from build123d import *

# Parameters (mm, degrees)
SKETCH_1_W             = 60
SKETCH_1_H             = 60
EXTRUDE_1_DEPTH        = 12
HOLE_WIZARD_M141_D     = 12
HOLE_WIZARD_M141_DEPTH = 12
SKETCH_12_R            = 4.5
CUT_EXTRUDE_1_DEPTH    = 13
SKETCH_13_R            = 7.5
CUT_EXTRUDE_2_DEPTH    = 9


with BuildPart() as part:
    # Эскиз1 → Бобышка-Вытянуть1 (new body)
    with BuildSketch(Plane(origin=(0, 0, 0), x_dir=(1, 0, 0), z_dir=(0, 1, 0))):
        Rectangle(SKETCH_1_W, SKETCH_1_H)
    extrude(amount=EXTRUDE_1_DEPTH)

    # Отверстие обработанное метчиком M141
    with Locations(Plane(origin=(0, 12, 0), x_dir=(1, 0, 0), z_dir=(0, 1, 0))):
        with Locations((0, 0)):
            Hole(HOLE_WIZARD_M141_D / 2, depth=HOLE_WIZARD_M141_DEPTH)

    # Эскиз12 → Вырез-Вытянуть1 (cut, through all)
    with BuildSketch(Plane(origin=(0, 12, 0), x_dir=(1, 0, 0), z_dir=(0, 1, 0))):
        with Locations(Location((-15, 15, 0), (0, 0, 270))):  # turned: the seam where the file's is
            Circle(SKETCH_12_R)
        with Locations(Location((15, 15, 0), (0, 0, 270))):  # turned: the seam where the file's is
            Circle(SKETCH_12_R)
        with Locations(Location((15, -15, 0), (0, 0, 270))):  # turned: the seam where the file's is
            Circle(SKETCH_12_R)
        with Locations(Location((-15, -15, 0), (0, 0, 270))):  # turned: the seam where the file's is
            Circle(SKETCH_12_R)
    extrude(amount=-CUT_EXTRUDE_1_DEPTH, mode=Mode.SUBTRACT)

    # Эскиз13 → Вырез-Вытянуть2 (cut)
    with BuildSketch(Plane(origin=(0, 12, 0), x_dir=(1, 0, 0), z_dir=(0, 1, 0))):
        with Locations(Location((-15, 15, 0), (0, 0, 270))):  # turned: the seam where the file's is
            Circle(SKETCH_13_R)
        with Locations(Location((15, 15, 0), (0, 0, 270))):  # turned: the seam where the file's is
            Circle(SKETCH_13_R)
        with Locations(Location((15, -15, 0), (0, 0, 270))):  # turned: the seam where the file's is
            Circle(SKETCH_13_R)
        with Locations(Location((-15, -15, 0), (0, 0, 270))):  # turned: the seam where the file's is
            Circle(SKETCH_13_R)
    extrude(amount=-CUT_EXTRUDE_2_DEPTH, mode=Mode.SUBTRACT)


solid = part.part
The model under review builds one solid part; all positions refer to its coordinate system, in mm. A direction names the side the tool comes from. Give positions to 0.01 mm unless a question says otherwise; leave off trailing zeros. Order: outer loops, then holes, each group sorted by start corner. A loop starts at its lowest first (then second) coordinate and runs counter-clockwise, first axis right, second up. Notation, with made-up numbers: M 66.25,-35.75 L 91.25,-35.75 A12 cw 91.25,-14.75 Z; hole C -2.5,18.25 d3. An arc over 180 degrees is marked long. Answer in a Markdown table with one row per item. Add a question column.
1. To check wall thickness, follow line 1 along X through (y, z) = (4.75, -15); line 2 along X through (y, z) = (1.8, 15); line 3 along Z through (x, y) = (-20, 10.5). State the ranges of each line that lie inside material, in increasing order.
2. Add section A-A on z = -15. State the section outline as (x, y) points, plus the area to 3 significant figures.
3. Mouldability with a two-part tool opening along X and no side actions: class faces 3 (the cylindrical face through (-11.96, 1.52, -18.32)), 4 (the flat face through (-30, 6, 0)), 5 (the flat face through (30, 6, 0)) as released by +X, released by -X, zero draft, split by the parting line, or undercut.
4. Machinability: for faces 1 (the cylindrical face through (15.33, 7.563, -22.493)), 2 (the flat face through (-7, 12, 0)), which of the approach directions +Z, -Z, +X, -X, +Y, -Y give a long, thin tool a straight path to every point of the face, cutting with its end or side? Answer none if there is none.
5. Add section D-D on z = 4. State the section outline as (x, y) points, plus the area to 3 significant figures.
6. For pin 1 Ø13.5 at (x, z) = (-15, -15) entering from +Y, flat-tipped, find the tip position at first contact; note if it passes through.
7. Add section B-B on y = 1.75. State the section outline as (x, z) points.
8. Add section C-C on x = 13. State the section outline as (y, z) points.
The answers:
| question | item | result |
|---|---|---|
| 1 | line 1 | -30 to -22.5, -7.5 to 7.5, 22.5 to 30 |
| 1 | line 2 | -30 to -19.5, -10.5 to 10.5, 19.5 to 30 |
| 1 | line 3 | -30 to -20.59, -9.41 to 9.41, 20.59 to 30 |
| 2 | outline | M -30,0 L -19.5,0 L -19.5,3 L -22.5,3 L -22.5,12 L -30,12 Z; M -10.5,0 L 10.5,0 L 10.5,3 L 7.5,3 L 7.5,12 L -7.5,12 L -7.5,3 L -10.5,3 Z; M 19.5,0 L 30,0 L 30,12 L 22.5,12 L 22.5,3 L 19.5,3 Z |
| 2 | area | 396 mm2 |
| 3 | face 3 | undercut |
| 3 | face 4 | released by -X |
| 3 | face 5 | released by +X |
| 4 | face 1 | +Y |
| 4 | face 2 | +Z, -Z, +X, -X, +Y |
| 5 | outline | M -30,0 L -4.47,0 L -4.47,12 L -30,12 Z; M 4.47,0 L 30,0 L 30,12 L 4.47,12 Z |
| 5 | area | 613 mm2 |
| 6 | pin 1 | y = 3 |
| 7 | outline | M -30,-30 L 30,-30 L 30,30 L -30,30 Z; hole C -15,-15 d9; hole C -15,15 d9; hole C 0,0 d12; hole C 15,-15 d9; hole C 15,15 d9 |
| 8 | outline | M 0,-30 L 12,-30 L 12,-22.23 L 3,-22.23 L 3,-19.03 L 0,-19.03 Z; M 0,-10.97 L 3,-10.97 L 3,-7.77 L 12,-7.77 L 12,7.77 L 3,7.77 L 3,10.97 L 0,10.97 Z; M 0,19.03 L 3,19.03 L 3,22.23 L 12,22.23 L 12,30 L 0,30 Z |
